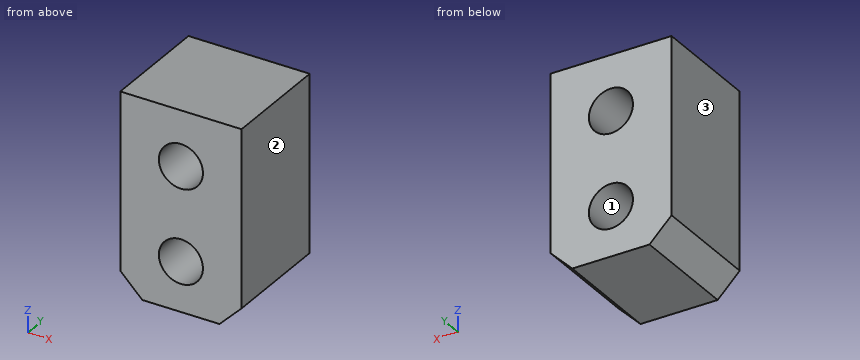
from build123d import *

# Parameters (mm, degrees)
SKETCH_1_W      = 22
SKETCH_1_H      = 36
SKETCH_1_R      = 4
EXTRUDE_1_DEPTH = 20
CHAMFER_1_SIZE  = 4


with BuildPart() as part:
    # 草图1 → 凸台-拉伸1 (new body)
    with BuildSketch(Plane(origin=(0, 0, 0), x_dir=(1, 0, 0), z_dir=(0, 1, 0))):
        with Locations((0.115789474, 0.4)):
            Rectangle(SKETCH_1_W, SKETCH_1_H)
        with Locations(Location((0.115789474, -7.6, 0), (0, 0, 270))):
            Circle(SKETCH_1_R, mode=Mode.SUBTRACT)
        with Locations(Location((0.115789474, 9.4, 0), (0, 0, 270))):
            Circle(SKETCH_1_R, mode=Mode.SUBTRACT)
    extrude(amount=EXTRUDE_1_DEPTH)

    # 倒角1
    chamfer_1_edges = [part.edges().sort_by_distance(p)[0] for p in [
        (-10.884210526, 10, -18.4),
        (11.115789474, 10, -18.4),
    ]]
    chamfer(chamfer_1_edges, length=CHAMFER_1_SIZE)


solid = part.part
CAD build for the part. Positions are in the model's coordinates, mm. Face numbers are marked on the shaded views. Round coordinates to 2 decimals unless told otherwise and drop trailing zeros. Loops run counter-clockwise (first coordinate to the right, second up) from the corner with the lowest first, then second, coordinate; pieces in that order, holes last.
(1) Cut at B-B (y = 3.5). Give the cut face in (x, z).
(2) Wall check: line 1 along Z through (x, y) = (0.25, 4.25); line 2 along X through (y, z) = (1.75, 7.5); line 3 along Z through (x, y) = (3, 11). Give the ranges that are in metal, low to high.
(3) Drop a flat-ended pin along its axis: pin 1 (13 mm diameter, centred on x = 0.12, z = 7.6, fed in from -Y). Give the stop position or say it passes through.
(4) Cut at C-C (z = 4). Give the cut face in (x, y).
(5) Cut at A-A (z = -9.4). Give the cut face in (x, y), plus the area to 3 significant figures.
(6) Two-plate mould, pull along X, no slides. Class the marked faces 1, 2 and 3: +X half, -X half, draft (parallel to the pull), parting line (faces both ways), or undercut.
Findings below:
1. outline: (-10.88, -14.4) - (-6.88, -18.4) - (7.12, -18.4) - (11.12, -14.4) - (11.12, 17.6) - (-10.88, 17.6) - close; hole circle Ø8 at (0.12, -9.4); hole circle Ø8 at (0.12, 7.6)
2. line 1: z = -18.4 to -13.4, -5.4 to 3.6, 11.6 to 17.6
2. line 2: x = -10.88 to -3.88, 4.11 to 11.12
2. line 3: z = -18.4 to -12.17, -6.63 to 4.83, 10.37 to 17.6
3. pin 1: stops at y = 0
4. outline: (-10.88, 0) - (-1.63, 0) - (-1.63, 20) - (-10.88, 20) - close; (1.86, 0) - (11.12, 0) - (11.12, 20) - (1.86, 20) - close
5. outline: (-10.88, 0) - (-3.88, 0) - (-3.88, 20) - (-10.88, 20) - close; (4.12, 0) - (11.12, 0) - (11.12, 20) - (4.12, 20) - close
5. area: 280 mm2
6. face 1: undercut
6. face 2: +X half
6. face 3: -X half
